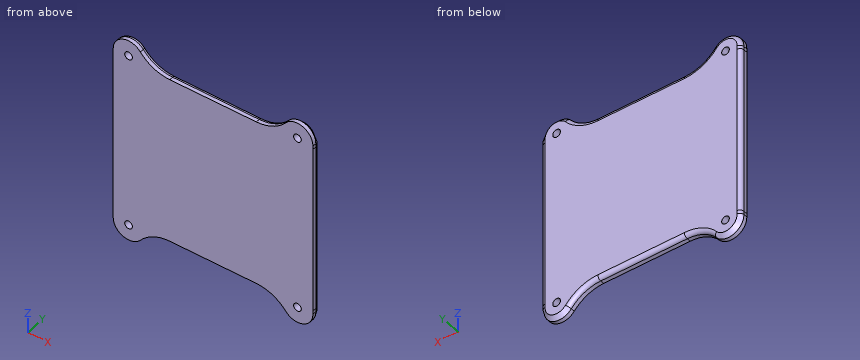
```python
from build123d import *

# Parameters (mm, degrees)
SKETCH1_R           = 1
BOSS_EXTRUDE1_DEPTH = 2
FILLET1_R           = 1


with BuildPart() as part:
    # Sketch1 → Boss-Extrude1 (new body)
    with BuildSketch(Plane(origin=(0, 20, 0), x_dir=(1, 0, 0), z_dir=(0, 1, 0))):
        with BuildLine():
            Line((11.276194705, 21.5), (-11.276194705, 21.5))
            ThreePointArc((-11.276194705, 21.5), (-15.501965979, 22.436730328), (-18.93605563, 25.071428571))
            ThreePointArc((-18.93605563, 25.071428571), (-23.440763365, 26.231514562), (-25.99700152, 22.345148936))
            ThreePointArc((-25.99700152, 22.345148936), (-25.989568255, 21.922542776), (-26, 21.5))
            Line((-26, 21.5), (-26, -21.5))
            ThreePointArc((-26, -21.5), (-25.989568255, -21.922542776), (-25.99700152, -22.345148936))
            ThreePointArc((-25.99700152, -22.345148936), (-23.440763365, -26.231514562), (-18.93605563, -25.071428571))
            ThreePointArc((-18.93605563, -25.071428571), (-15.501965979, -22.436730328), (-11.276194705, -21.5))
            Line((-11.276194705, -21.5), (11.276194705, -21.5))
            ThreePointArc((11.276194705, -21.5), (15.501965979, -22.436730328), (18.93605563, -25.071428571))
            ThreePointArc((18.93605563, -25.071428571), (23.440763365, -26.231514562), (25.99700152, -22.345148936))
            ThreePointArc((25.99700152, -22.345148936), (25.989568255, -21.922542776), (26, -21.5))
            Line((26, -21.5), (26, 21.5))
            ThreePointArc((26, 21.5), (25.989568255, 21.922542776), (25.99700152, 22.345148936))
            ThreePointArc((25.99700152, 22.345148936), (23.440763365, 26.231514562), (18.93605563, 25.071428571))
            ThreePointArc((18.93605563, 25.071428571), (15.501965979, 22.436730328), (11.276194705, 21.5))
        make_face()
        with Locations(Location((-22, -22.5, 0), (0, 0, 270))):
            Circle(SKETCH1_R, mode=Mode.SUBTRACT)
        with Locations(Location((22, -22.5, 0), (0, 0, 270))):
            Circle(SKETCH1_R, mode=Mode.SUBTRACT)
        with Locations(Location((22, 22.5, 0), (0, 0, 270))):
            Circle(SKETCH1_R, mode=Mode.SUBTRACT)
        with Locations(Location((-22, 22.5, 0), (0, 0, 270))):
            Circle(SKETCH1_R, mode=Mode.SUBTRACT)
    extrude(amount=BOSS_EXTRUDE1_DEPTH)

    # Fillet1
    # the kernel refuses this fillet: 1 mm, written as the material it takes off along each edge
    with BuildSketch(Plane(origin=(-11.276194705, 22, -31.5), x_dir=(0, 0, 1), z_dir=(1, 0, 0))) as fillet1_piece_1:
        with BuildLine():
            CenterArc((10 + FILLET1_R, FILLET1_R), FILLET1_R, 180, 90)
            Line((10 + FILLET1_R, 0), (10, 0))
            Line((10, 0), (10, FILLET1_R))
        make_face()
    revolve(axis=Axis((-11.276194705, 22, -31.5), (0, -1, 0)), revolution_arc=49.994799115, mode=Mode.SUBTRACT)
    with BuildSketch(Plane(origin=(-22, 22, -22.5), x_dir=(0.7659860924831153, 0, -0.6428571428571425), z_dir=(0.6428571428571425, 0, 0.7659860924831153))) as fillet1_piece_2:
        with BuildLine():
            CenterArc((4 - FILLET1_R, -FILLET1_R), FILLET1_R, 0, 90)
            Line((4 - FILLET1_R, 0), (4, 0))
            Line((4, 0), (4, -FILLET1_R))
        make_face()
    revolve(axis=Axis((-22, 22, -22.5), (0, 1, 0)), revolution_arc=142.21343163, mode=Mode.SUBTRACT)
    with BuildSketch(Plane(origin=(-35.989505319, 22, -21.958021275), x_dir=(0.999250379905618, 0, -0.03871276609179466), z_dir=(-0.03871276609179466, 0, -0.999250379905618))) as fillet1_piece_3:
        with BuildLine():
            CenterArc((10 + FILLET1_R, FILLET1_R), FILLET1_R, 180, 90)
            Line((10 + FILLET1_R, 0), (10, 0))
            Line((10, 0), (10, FILLET1_R))
        make_face()
    revolve(axis=Axis((-35.989505319, 22, -21.958021275), (0, -1, 0)), revolution_arc=19.167781067, mode=Mode.SUBTRACT)
    with BuildSketch(Plane(origin=(-26, 22, -24), x_dir=(0, -1, 0), z_dir=(0, 0, 1)), Plane(origin=(26, 22, 24), x_dir=(0, -1, 0), z_dir=(0, 0, -1))) as fillet1_piece_4:
        with BuildLine():
            CenterArc((FILLET1_R, FILLET1_R), FILLET1_R, 180, 90)
            Line((0, FILLET1_R), (0, 0))
            Line((0, 0), (FILLET1_R, 0))
        make_face()
    extrude(amount=48, mode=Mode.SUBTRACT)
    with BuildSketch(Plane(origin=(-35.989505319, 22, 21.958021275), x_dir=(0.9565638665427638, 0, -0.2915228451163944), z_dir=(-0.2915228451163944, 0, -0.9565638665427638))) as fillet1_piece_5:
        with BuildLine():
            CenterArc((10 + FILLET1_R, FILLET1_R), FILLET1_R, 180, 90)
            Line((10 + FILLET1_R, 0), (10, 0))
            Line((10, 0), (10, FILLET1_R))
        make_face()
    revolve(axis=Axis((-35.989505319, 22, 21.958021275), (0, -1, 0)), revolution_arc=19.167781067, mode=Mode.SUBTRACT)
    with BuildSketch(Plane(origin=(-22, 22, 22.5), x_dir=(-0.9992503799056173, 0, -0.03871276609181696), z_dir=(0.03871276609181696, 0, -0.9992503799056173))) as fillet1_piece_6:
        with BuildLine():
            CenterArc((4 - FILLET1_R, -FILLET1_R), FILLET1_R, 0, 90)
            Line((4 - FILLET1_R, 0), (4, 0))
            Line((4, 0), (4, -FILLET1_R))
        make_face()
    revolve(axis=Axis((-22, 22, 22.5), (0, 1, 0)), revolution_arc=142.21343163, mode=Mode.SUBTRACT)
    with BuildSketch(Plane(origin=(-11.276194705, 22, 31.5), x_dir=(-0.7659860924831162, 0, -0.6428571428571414), z_dir=(-0.6428571428571414, 0, 0.7659860924831162))) as fillet1_piece_7:
        with BuildLine():
            CenterArc((10 + FILLET1_R, FILLET1_R), FILLET1_R, 180, 90)
            Line((10 + FILLET1_R, 0), (10, 0))
            Line((10, 0), (10, FILLET1_R))
        make_face()
    revolve(axis=Axis((-11.276194705, 22, 31.5), (0, -1, 0)), revolution_arc=49.994799115, mode=Mode.SUBTRACT)
    with BuildSketch(Plane(origin=(-11.276194705, 22, 21.5), x_dir=(0, -1, 0), z_dir=(1, 0, 0)), Plane(origin=(11.276194705, 22, -21.5), x_dir=(0, -1, 0), z_dir=(-1, 0, 0))) as fillet1_piece_8:
        with BuildLine():
            CenterArc((FILLET1_R, FILLET1_R), FILLET1_R, 180, 90)
            Line((0, FILLET1_R), (0, 0))
            Line((0, 0), (FILLET1_R, 0))
        make_face()
    extrude(amount=22.55238941, mode=Mode.SUBTRACT)
    with BuildSketch(Plane(origin=(11.276194705, 22, 31.5), x_dir=(0, 0, -1), z_dir=(-1, 0, 0))) as fillet1_piece_9:
        with BuildLine():
            CenterArc((10 + FILLET1_R, FILLET1_R), FILLET1_R, 180, 90)
            Line((10 + FILLET1_R, 0), (10, 0))
            Line((10, 0), (10, FILLET1_R))
        make_face()
    revolve(axis=Axis((11.276194705, 22, 31.5), (0, -1, 0)), revolution_arc=49.994799115, mode=Mode.SUBTRACT)
    with BuildSketch(Plane(origin=(22, 22, 22.5), x_dir=(-0.7659860924831153, 0, 0.6428571428571425), z_dir=(-0.6428571428571425, 0, -0.7659860924831153))) as fillet1_piece_10:
        with BuildLine():
            CenterArc((4 - FILLET1_R, -FILLET1_R), FILLET1_R, 0, 90)
            Line((4 - FILLET1_R, 0), (4, 0))
            Line((4, 0), (4, -FILLET1_R))
        make_face()
    revolve(axis=Axis((22, 22, 22.5), (0, 1, 0)), revolution_arc=142.21343163, mode=Mode.SUBTRACT)
    with BuildSketch(Plane(origin=(11.276194705, 22, -31.5), x_dir=(0.7659860924831151, 0, 0.6428571428571426), z_dir=(0.6428571428571426, 0, -0.7659860924831151))) as fillet1_piece_11:
        with BuildLine():
            CenterArc((10 + FILLET1_R, FILLET1_R), FILLET1_R, 180, 90)
            Line((10 + FILLET1_R, 0), (10, 0))
            Line((10, 0), (10, FILLET1_R))
        make_face()
    revolve(axis=Axis((11.276194705, 22, -31.5), (0, -1, 0)), revolution_arc=49.994799115, mode=Mode.SUBTRACT)
    with BuildSketch(Plane(origin=(35.989505319, 22, 21.958021275), x_dir=(-0.999250379905617, 0, 0.03871276609181962), z_dir=(0.03871276609181962, 0, 0.999250379905617))) as fillet1_piece_12:
        with BuildLine():
            CenterArc((10 + FILLET1_R, FILLET1_R), FILLET1_R, 180, 90)
            Line((10 + FILLET1_R, 0), (10, 0))
            Line((10, 0), (10, FILLET1_R))
        make_face()
    revolve(axis=Axis((35.989505319, 22, 21.958021275), (0, -1, 0)), revolution_arc=19.167781067, mode=Mode.SUBTRACT)
    with BuildSketch(Plane(origin=(35.989505319, 22, -21.958021275), x_dir=(-0.9565638665427474, 0, 0.2915228451164487), z_dir=(0.2915228451164487, 0, 0.9565638665427474))) as fillet1_piece_13:
        with BuildLine():
            CenterArc((10 + FILLET1_R, FILLET1_R), FILLET1_R, 180, 90)
            Line((10 + FILLET1_R, 0), (10, 0))
            Line((10, 0), (10, FILLET1_R))
        make_face()
    revolve(axis=Axis((35.989505319, 22, -21.958021275), (0, -1, 0)), revolution_arc=19.167781067, mode=Mode.SUBTRACT)
    with BuildSketch(Plane(origin=(22, 22, -22.5), x_dir=(0.9992503799056174, 0, 0.038712766091811596), z_dir=(-0.038712766091811596, 0, 0.9992503799056174))) as fillet1_piece_14:
        with BuildLine():
            CenterArc((4 - FILLET1_R, -FILLET1_R), FILLET1_R, 0, 90)
            Line((4 - FILLET1_R, 0), (4, 0))
            Line((4, 0), (4, -FILLET1_R))
        make_face()
    revolve(axis=Axis((22, 22, -22.5), (0, 1, 0)), revolution_arc=142.21343163, mode=Mode.SUBTRACT)


solid = part.part
```
Input: part model. Units: mm. Frame: model coordinates. Give positions to 0.01 mm unless a question says otherwise; leave off trailing zeros. Loops run counter-clockwise (first coordinate to the right, second up) from the corner with the lowest first, then second, coordinate; pieces in that order, holes last.
1) Contact query for flat-ended pins moving along their axis: pin 1 (1.1 mm diameter, centred on x = 5.5, y = 20.5, fed in from +Z); pin 2 (1.6 mm diameter, centred on x = -22, z = -22.5, fed in from +Y); pin 3 (0.5 mm diameter, centred on x = 1.5, y = 20.5, fed in from -Z). Output: stop coordinate, or through.
A:
pin 1: stops at z = 21.5
pin 2: passes through
pin 3: stops at z = -21.5
2) Line query: L1, parallel to X at y = 21.1, z = -22.5; L2, parallel to X at y = 21.2, z = 7; L3, parallel to X at y = 21.6, z = 22.5. Output: solid intervals per line, ascending.
A:
L1: x = -25.99 to -23, -21 to -15.65, 15.65 to 21, 23 to 25.99
L2: x = -25.98 to 25.98
L3: x = -25.8 to -23, -21 to -16.08, 16.08 to 21, 23 to 25.8
3) Section query B-B on y = 20.5. Return the cut outline in (x, z), and give its area (3 significant figures).
A:
outline: (-26, -22.35) arc R4 ccw to (-18.94, -25.07) arc R10 cw to (-11.28, -21.5) - (11.28, -21.5) arc R10 cw to (18.94, -25.07) arc R4 ccw to (26, -22.35) arc R10 cw to (26, -21.5) - (26, 21.5) arc R10 cw to (26, 22.35) arc R4 ccw to (18.94, 25.07) arc R10 cw to (11.28, 21.5) - (-11.28, 21.5) arc R10 cw to (-18.94, 25.07) arc R4 ccw to (-26, 22.35) arc R10 cw to (-26, 21.5) - (-26, -21.5) arc R10 cw to start; hole circle Ø2 at (-22, -22.5); hole circle Ø2 at (-22, 22.5); hole circle Ø2 at (22, -22.5); hole circle Ø2 at (22, 22.5)
area: 2,380 mm2
